Can you work these out from the model? Positions are in its coordinate system, mm. A direction names the side the tool comes from. Give positions to 0.01 mm unless a question says otherwise; leave off trailing zeros. Answer as CSV lines item,"result".
Autodesk Inventor part; units mm, degrees
ref_plane "Work Plane2" through (0, 0, 0) normal (-0.7071, 0, 0.7071) x (0, 1, 0)
ref_plane "Work Plane3" through (0, 1, 0) normal (0, -1, 0) x (1, 0, 0)
ref_plane "YZ Plane" through (0, 0, 0) normal (1, 0, 0) x (0, 1, 0)
sketch "Sketch1" plane through (0, 0, 0) normal (0, 1, 0) x (-1, 0, 0)
  line L0 (0, 0) -> (25, 0)
  line L1 (25, 0) -> (25, -25)
  line L2 (25, -25) -> (0, -25)
  line L3 (0, -25) -> (0, 0)
  circle A0 centre (12.5, -12.5) radius 17.6777
  circle A1 centre (12.5, -12.5) radius 21.86
  dimension "d0" = 25
  dimension "d1" = 25
  dimension "d2" = 43.72
extrude "Extrusion1" add sketch "Sketch1" along normal blind 1 contours L0 L1 L2 L3
ref_plane "Work Plane2" through (0, 0, 0) normal (-0.7071, 0, 0.7071) x (0, 1, 0)
sketch "Sketch3" plane through (0, 0, 0) normal (-0.7071, 0, 0.7071) x (0, 1, 0)
  line L0 (1, 0) -> (1, 17.6777)
  line L1 (1, 17.6777) -> (1, 35.3553)
  line L2 (1, 17.6777) -> (7.5, 17.6777) construction
  arc A0 (1, 0) -> (1, 35.3553) centre (-19.7885, 17.6777) ccw construction
  circle A1 centre (-19.7885, 17.6777) radius 27.375 construction
  circle A2 centre (-19.7885, 17.6777) radius 27.375
  circle A3 centre (-19.7885, 17.6777) radius 27.875
  line L3 (7.5, 17.6777) -> (8.0865, 17.6777)
  line L4 (-19.7885, 45.0527) -> (-19.7885, 45.5527)
  line L5 (-19.7885, 17.6777) -> (-5.3263, 17.6777)
  line L6 (-19.7885, 17.6777) -> (-19.7885, 45.0527)
  point P0 (0, 0)
  point P1 (7.5865, 17.6777)
  dimension "d10" = 6.5
  dimension "d11" = 54.75
  dimension "d12" = 55.75
revolve "Revolution1" add sketch "Sketch3" angle 360 about axis through (-12.5, -19.7885, -12.5) along (0, 1, 0) picked at (-9.7302, 43.3292) contours A2 L4 A3 L3
ref_plane "Work Plane3" through (0, 1, 0) normal (0, -1, 0) x (1, 0, 0)
sketch "Sketch4" plane through (0, 1, 0) normal (0, -1, 0) x (1, 0, 0)
  line L0 (0, -25) -> (-25, -25) construction
  line L1 (0, 0) -> (0, -25) construction
  line L2 (-25, 0) -> (0, 0) construction
  line L3 (-25, -25) -> (-25, 0) construction
  line L4 (-25, 0) -> (-23, 0) construction
  line L5 (-23, 0) -> (-23, -2) construction
  line L6 (-23, -2) -> (-25, -2) construction
  line L7 (-25, -2) -> (-25, 0) construction
  line L8 (0, 0) -> (-2, 0) construction
  line L9 (-2, 0) -> (-2, -2) construction
  line L10 (-2, -2) -> (0, -2) construction
  line L11 (0, -2) -> (0, 0) construction
  circle A0 centre (-23, -2) radius 1 construction
  circle A1 centre (-23, -2) radius 1
  circle A2 centre (-23, -2) radius 2
  circle A3 centre (-2, -2) radius 1
  circle A4 centre (-2, -2) radius 2
  line L12 (-25, 0) -> (-23, 0) construction
  line L13 (-23, 0) -> (-23, -14.5) construction
  line L14 (-23, -14.5) -> (-25, -14.5) construction
  line L15 (-25, -14.5) -> (-25, 0) construction
  line L16 (0, 0) -> (-2, 0) construction
  line L17 (-2, 0) -> (-2, -14.5) construction
  line L18 (-2, -14.5) -> (0, -14.5) construction
  line L19 (0, -14.5) -> (0, 0) construction
  circle A5 centre (-23, -14.5) radius 1
  circle A6 centre (-2, -14.5) radius 1
  circle A7 centre (-23, -14.5) radius 2
  circle A8 centre (-2, -14.5) radius 2
  dimension "d15" = 2
  dimension "d16" = 2
  dimension "d17" = 2
  dimension "d18" = 2
  dimension "d19" = 2
  dimension "d20" = 4
  dimension "d21" = 2
  dimension "d22" = 4
  dimension "d23" = 2
  dimension "d24" = 14.5
  dimension "d25" = 2
  dimension "d26" = 14.5
  dimension "d27" = 2
  dimension "d28" = 2
  dimension "d29" = 4
  dimension "d30" = 4
extrude "Extrusion2" add sketch "Sketch4" against normal up to surface
sketch "Sketch5" plane through (0, 0, 0) normal (0, -1, 0) x (1, 0, 0)
  line L0 (0, -25) -> (-25, -25) construction
  line L1 (0, 0) -> (0, -25) construction
  line L2 (-25, 0) -> (0, 0) construction
  line L3 (-25, -25) -> (-25, 0) construction
  line L4 (-12.5, 0) -> (-12.5, -14.5) construction
  circle A0 centre (-12.5, -14.5) radius 4.5
  dimension "d33" = 14.5
  dimension "d34" = 9
extrude "Extrusion3" cut sketch "Sketch5" against normal blind 10
sketch "Sketch6" plane through (0, 0, 0) normal (0, -1, 0) x (1, 0, 0)
  circle A0 centre (-12.5, -14.5) radius 4.5
  line L0 (0, -25) -> (-25, -25)
  line L1 (0, 0) -> (0, -25)
  line L2 (-25, 0) -> (0, 0)
  line L3 (-25, -25) -> (-25, 0)
extrude "Extrusion4" cut sketch "Sketch6" against normal blind 1
properties part number "Ball"
1) Which directions (+Z, -Z, +X, -X, +Y, -Y) give clear straight access to the entire face, cutting with the end or side of a thin tool? Please do faces 1 (the cylindrical face through (-3.998, 2.975, -14.412)), 2 (the cylindrical face through (-16.996, 7.381, -14.302)).
Answer block:
face 1,"-Y"
face 2,"+Y, -Y"
2) I'm going to push flat-ended pins straight in: P1, Ø2.5, axis at x = -2, z = -14.5, coming from the +Y side; P2, Ø1.5, axis at x = -6.5, y = -8, coming from the -Z side; P3, Ø1.6, axis at x = -23, z = -14.5, coming from the -Y side; P4, Ø5.5, axis at x = -12.5, z = -14.5, coming from the +Y side. Where does each tip first touch, or does it pass through?
Answer block:
P1,"y = 6.44"
P2,"z = -37.43"
P3,"y = 5.06"
P4,"through"
3) If we mould it in two halves opening along Z, with no side actions, what happens to faces 3 (the cylindrical face through (-22.077, 2.292, -3.774)), 4 (the flat face through (-11, -19.788, -40))? For each: +Z half, -Z half, draft (parallel to the pull), parting line (faces both ways), or undercut.
Answer block:
face 3,"undercut"
face 4,"draft"
4) I need wall thicknesses on line 1 along Z through (x, y) = (-2, 1.7); line 2 along X through (y, z) = (3.2, -2); line 3 along Z through (x, y) = (-23, 2.8). Which ranges of each line are inside material? Lowest first, please. Write a range as [from, to].
Answer block:
line 1,"[-26.82, -25.82], [-16.5, -15.5], [-13.5, -12.5], [-4, -3], [-1, 0], [0.82, 1.82]"
line 2,"[-24.26, -23.02], [-22, -21], [-4, -3], [-1.98, -0.74]"
line 3,"[-25.01, -23.85], [-16.5, -15.5], [-13.5, -12.5], [-4, -3], [-1.15, 0.01]"
